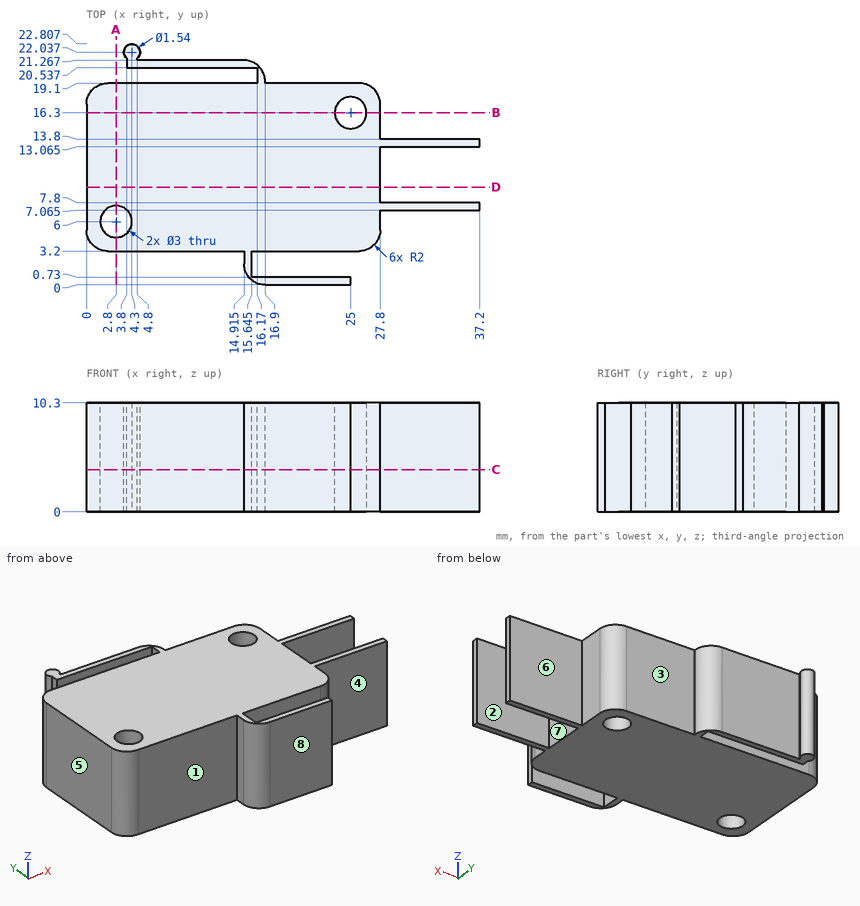
For this review, use the dimensioned drawing (mm, ordinates from the lowest corner) and the shaded views. A direction names the side the tool comes from. Coordinates: 2 decimals unless noted, no trailing zeros. Order: outer loops, then holes, each group sorted by start corner. A loop starts at its lowest first (then second) coordinate and runs counter-clockwise, first axis right, second up. Notation, with made-up numbers: (-35, 2) -> (23, 2) arc R25 cw to (23, 31) -> close; hole circle Ø4 at (45, -1). An arc over 180 degrees is marked (long way). One line per item, written item: value. Start each with the question number.
Q1. For probe 1 along Y at (x, z) = (2.8, 3.75); probe 2 along Y at (x, z) = (14, 4.5); probe 3 along X at (y, z) = (16.3, 4), list the stretches that pass through material, from the lowest coordinate up.
Q2. Take a section at C-C, the plane z = 4. Give the number of separate pieces and of enclosed holes in the cut face, then the cut area to 3 significant figures.
Q3. Tool access review of the marked faces 1, 2, 3 and 4: name each direction out of +Z, -Z, +X, -X, +Y, -Y from which nothing blocks a thin tool from reaching the whole face with its end or side.
Q4. Take a section at D-D, the plane y = 9.25. State the section outline as (x, z) points.
Q5. Insertion check: pin 1 Ø4.5 at (x, z) = (32.5, 3) entering from -Y (1 decimal); pin 2 Ø4 at (x, z) = (14, 1) entering from +Y; pin 3 Ø2.5 at (y, z) = (10.5, 5) entering from +X; pin 4 Ø2.5 at (x, y) = (2.8, 6) entering from -Z. Each pin has a flat end and moves straight along its axis. Give the tip position at first contact, or say it passes through.
Q6. Take a section at A-A, the plane x = 2.8. State the section outline as (y, z) points, then the cut area to 3 significant figures.
Q7. Take a section at B-B, the plane y = 16.3. State the section outline as (x, z) points.
Q8. Mouldability with a two-part tool opening along Y and no side actions: class the marked faces 5, 6, 7 and 8 as pulls with the +Y half, pulls with the -Y half, needs draft (parallel to the pull), parting line crosses it, or undercut.
Values follow:
1. probe 1: y = 3.2 to 4.5, 7.5 to 19.1
1. probe 2: y = 3.2 to 19.1, 20.54 to 21.27
1. probe 3: x = 0 to 23.5, 26.5 to 27.8
2. separate pieces: 1
2. enclosed holes: 2
2. area: 458 mm2
3. face 1: +Z, -Z, -X, -Y
3. face 2: +Z, -Z, +X
3. face 3: +Z, -Z, +X, +Y
3. face 4: +Z, -Z, +X, -Y
4. outline: (0, 0) -> (27.8, 0) -> (27.8, 10.3) -> (0, 10.3) -> close
5. pin 1: stops at y = 7.1
5. pin 2: stops at y = 21.27
5. pin 3: stops at x = 27.8
5. pin 4: passes through
6. outline: (3.2, 0) -> (4.5, 0) -> (4.5, 10.3) -> (3.2, 10.3) -> close; (7.5, 0) -> (19.1, 0) -> (19.1, 10.3) -> (7.5, 10.3) -> close
6. area: 133 mm2
7. outline: (0, 0) -> (23.5, 0) -> (23.5, 10.3) -> (0, 10.3) -> close; (26.5, 0) -> (27.8, 0) -> (27.8, 10.3) -> (26.5, 10.3) -> close
8. face 5: needs draft
8. face 6: pulls with the +Y half
8. face 7: undercut
8. face 8: pulls with the -Y half
